Read the model definition and answer for the solid it produces. Units are mm, in the model's axes. A direction names the side the tool comes from. Coordinates: 2 decimals unless noted, no trailing zeros. Write each loop counter-clockwise with the first axis right and the second up, starting at its lowest first coordinate (ties: lowest second). Pieces come first, ordered by that corner, then holes.
Item 1: Each of these flat-tipped pins is pushed along its axis until it touches: P1, Ø4.5, axis at x = -9, z = -9.5, coming from the -Y side; P2, Ø18, axis at x = -47, z = -8, coming from the -Y side; P3, Ø10, axis at x = -26.5, y = 9.5, coming from the +Z side; P4, Ø2, axis at y = 11.5, z = -3, coming from the -X side. Where does it stop, or does it pass through?
Item 2: Straight lines are drawn through the part: probe 1 along Y at (x, z) = (-68, 11); probe 2 along Z at (x, y) = (7, 49.5); probe 3 along Y at (x, z) = (16, 2.5). For each, find the intervals that lie inside material, in ascending order.
Item 3: A tool of negligible diameter and unlimited length cuts with its end or side. For faces 4 (the face through (23, 30, -29)), 5 (the face through (-25, 47, 0)), 6 (the face through (-61.466, 57.479, -10.082)), 7 (the face through (7.5, 46.5, 10.7)), 8 (the face through (20, 6, 0)), from which of +Z, -Z, +X, -X, +Y, -Y can it reach the whole face along a straight path? Write none if from no direction.
Item 4: Determine the mould class of faces 1 (the face through (-51.5, 62, -14)), 2 (the face through (1, 80, 28)), 3 (the face through (23, 1, -19)) for opening direction Z: released by +Z, released by -Z, zero draft, split by the parting line, or undercut.
Item 5: Section A-A (x = -16.5) is taken. Give the vertices of the cut face in (y, z) (3 decimals).
Item 6: Section C-C (y = 39) is taken. Give the vertices of the cut face in (x, z) (3 decimals), then the cut area to 3 significant figures.
Item 7: Section D-D (x = 81) is taken. Give the vertices of the cut face in (y, z).
Item 8: Section B-B (z = 19) is taken. Give the vertices of the cut face in (x, y).
from build123d import *

# Parameters (mm, degrees)
BOSS_EXTRUDE1_DEPTH            = 30
BOSS_EXTRUDE1_DEPTH_BACK       = 30
CUT_REVOLVE2_START             = 59
CUT_REVOLVE2_DEPTH             = 7
CUT_REVOLVE2_START_2           = 56
CUT_REVOLVE2_2_DEPTH           = 3
CUT_EXTRUDE1_DEPTH             = 22.615
CUT_EXTRUDE2_REACH             = 143.287
CUT_EXTRUDE2_DIRECTION_2_DEPTH = 142.286942072
FILLET5_R                      = 5
FILLET6_R                      = 5
SKETCH7_W                      = 18.23
SKETCH7_H                      = 1.85
CUT_EXTRUDE3_DEPTH             = 17.32
SKETCH8_W                      = 20
SKETCH8_H                      = 24.63
CUT_EXTRUDE4_DEPTH             = 15.3
CUT_EXTRUDE5_REACH             = 133.385
SKETCH10_R                     = 1
SKETCH12_R                     = 2.5
CUT_EXTRUDE6_DEPTH             = 10.5
CUT_EXTRUDE7_REACH             = 133.385
SKETCH13_R                     = 1
SKETCH14_R                     = 2.5
CUT_EXTRUDE8_DEPTH             = 34.5


# Read off the part's stored shape, not the designer's step: Cut-Revolve2
with BuildPart() as part:
    # Sketch1 → Boss-Extrude1 (new, two sides: drawn at the far end of the back side and taken through both)
    with BuildSketch(Plane.XY.offset(-BOSS_EXTRUDE1_DEPTH_BACK)):
        Polygon((-25, 0), (-25, 56), (-99, 56), (-99, 81), (99, 81), (99, 56), (25, 56), (25, 0), align=None)
    extrude(amount=BOSS_EXTRUDE1_DEPTH + BOSS_EXTRUDE1_DEPTH_BACK)

    # Cut-Revolve2 outline → Cut-Revolve2 (cut)
    with BuildSketch(Plane(origin=(0, 0, 0), x_dir=(1, 0, 0), z_dir=(0, 1, 0)).offset(CUT_REVOLVE2_START)):
        with BuildLine():
            ThreePointArc((-37.5, -6), (-43.043277195, -2.296100594), (-41.742640687, 4.242640687))
            Line((-41.742640687, 4.242640687), (-61.54163056, 24.04163056))
            ThreePointArc((-61.54163056, 24.04163056), (-71.129711609, -5.004247907), (-53.5, -30))
            Line((-53.5, -30), (-37.5, -30))
            Line((-37.5, -30), (-37.5, -6))
        make_face()
    cut_revolve2 = extrude(amount=CUT_REVOLVE2_DEPTH, mode=Mode.SUBTRACT)

    # Cut-Revolve2 2 outline → Cut-Revolve2 2 (cut)
    with BuildSketch(Plane(origin=(0, 0, 0), x_dir=(1, 0, 0), z_dir=(0, 1, 0)).offset(CUT_REVOLVE2_START_2)):
        with BuildLine():
            Line((-37.5, -26), (-37.5, -14))
            ThreePointArc((-37.5, -14), (-50.434313455, -5.357568053), (-47.399494937, 9.899494937))
            Line((-47.399494937, 9.899494937), (-55.884776311, 18.384776311))
            ThreePointArc((-55.884776311, 18.384776311), (-61.520867845, -9.949769241), (-37.5, -26))
        make_face()
    cut_revolve2_2 = extrude(amount=CUT_REVOLVE2_2_DEPTH, mode=Mode.SUBTRACT)

    # Sketch4 → Cut-Extrude1 (cut)
    with BuildSketch(Plane.ZY.offset(25)):
        Polygon((12.315, 12.5), (-12.315, 12.5), (-12.315, 44.5), (-6.965, 44.5), (-6.965, 45.65), (7.015, 45.65), (7.015, 44.5), (12.315, 44.5), align=None)
    cut_extrude1 = extrude(amount=-CUT_EXTRUDE1_DEPTH, mode=Mode.SUBTRACT)

    # Mirror1: Cut-Extrude1 across plane
    add(cut_extrude1.mirror(Plane.ZY), mode=Mode.SUBTRACT)

    # Sketch5 → Cut-Extrude2 (cut, up to next)
    with BuildSketch(Plane.XY.offset(30), mode=Mode.PRIVATE) as cut_extrude2_sk1:
        Polygon((-63.5, 56), (-37.5, 56), (-37.5, 66), (-71.5, 66), (-71.5, 59), (-63.5, 59), align=None)
    cut_extrude2_tool1 = extrude(cut_extrude2_sk1.sketch, amount=-CUT_EXTRUDE2_REACH, mode=Mode.PRIVATE) & part.part
    cut_extrude2 = cut_extrude2_tool1.solids().sort_by_distance((-53.512658, 61.265823, 30))[0]
    add(cut_extrude2, mode=Mode.SUBTRACT)

    # Sketch5 → Cut-Extrude2 direction 2 (cut)
    with BuildSketch(Plane.XY.offset(30)):
        Polygon((-63.5, 56), (-37.5, 56), (-37.5, 66), (-71.5, 66), (-71.5, 59), (-63.5, 59), align=None)
    cut_extrude2_direction_2 = extrude(amount=CUT_EXTRUDE2_DIRECTION_2_DEPTH, mode=Mode.SUBTRACT)

    # Mirror4: Cut-Revolve2, Cut-Revolve2 2 across plane
    add(cut_revolve2.mirror(Plane.ZY), mode=Mode.SUBTRACT)
    add(cut_revolve2_2.mirror(Plane.ZY), mode=Mode.SUBTRACT)

    # Mirror2: Cut-Extrude2, Cut-Extrude2 direction 2 across plane
    add(cut_extrude2.mirror(Plane.ZY), mode=Mode.SUBTRACT)
    add(cut_extrude2_direction_2.mirror(Plane.ZY), mode=Mode.SUBTRACT)

    # Fillet5
    fillet5_edges = [part.edges().sort_by_distance(p)[0] for p in [
        (-99, 81, 0),
        (99, 81, 0),
        (0, 81, -30),
        (0, 81, 30),
    ]]
    fillet(fillet5_edges, radius=FILLET5_R)

    # Fillet6
    fillet6_edges = [part.edges().sort_by_distance(p)[0] for p in [
        (-25, 0, 0),
        (-99, 56, 0),
        (99, 56, 0),
        (25, 0, 0),
        (0, 0, 30),
        (25, 28, 30),
        (-25, 28, 30),
        (-25, 28, -30),
        (0, 0, -30),
        (25, 28, -30),
    ]]
    fillet(fillet6_edges, radius=FILLET6_R)

    # Sketch7 → Cut-Extrude3 (cut)
    with BuildSketch(Plane.ZY.offset(25)):
        with Locations((0, 11.575)):
            Rectangle(SKETCH7_W, SKETCH7_H)
    cut_extrude3 = extrude(amount=-CUT_EXTRUDE3_DEPTH, mode=Mode.SUBTRACT)

    # Mirror5: Cut-Extrude3 across plane
    add(cut_extrude3.mirror(Plane.ZY), mode=Mode.SUBTRACT)

    # Sketch8 → Cut-Extrude4 (cut)
    with BuildSketch(Plane.XZ):
        with Locations((-30, 0)):
            Rectangle(SKETCH8_W, SKETCH8_H)
        with Locations((30, 0)):
            Rectangle(SKETCH8_W, SKETCH8_H)
    extrude(amount=-CUT_EXTRUDE4_DEPTH, mode=Mode.SUBTRACT)

    # Sketch10 → Cut-Extrude5 (cut, up to next)
    with BuildSketch(Plane(origin=(0, 0, 0), x_dir=(-1, 0, 0), z_dir=(0, -1, 0)), mode=Mode.PRIVATE) as cut_extrude5_sk1:
        with Locations(Location((4.785, -10.165, 0), (0, 0, 90))):
            Circle(SKETCH10_R)
    cut_extrude5_tool1 = extrude(cut_extrude5_sk1.sketch, amount=-CUT_EXTRUDE5_REACH, mode=Mode.PRIVATE) & part.part
    # Sketch10 → Cut-Extrude5 (cut, up to next)
    with BuildSketch(Plane(origin=(0, 0, 0), x_dir=(-1, 0, 0), z_dir=(0, -1, 0)), mode=Mode.PRIVATE) as cut_extrude5_sk2:
        with Locations(Location((4.785, 10.165, 0), (0, 0, 180))):
            Circle(SKETCH10_R)
    cut_extrude5_tool2 = extrude(cut_extrude5_sk2.sketch, amount=-CUT_EXTRUDE5_REACH, mode=Mode.PRIVATE) & part.part
    # Sketch10 → Cut-Extrude5 (cut, up to next)
    with BuildSketch(Plane(origin=(0, 0, 0), x_dir=(-1, 0, 0), z_dir=(0, -1, 0)), mode=Mode.PRIVATE) as cut_extrude5_sk3:
        with Locations(Location((-4.785, 10.165, 0), (0, 0, 90))):
            Circle(SKETCH10_R)
    cut_extrude5_tool3 = extrude(cut_extrude5_sk3.sketch, amount=-CUT_EXTRUDE5_REACH, mode=Mode.PRIVATE) & part.part
    # Sketch10 → Cut-Extrude5 (cut, up to next)
    with BuildSketch(Plane(origin=(0, 0, 0), x_dir=(-1, 0, 0), z_dir=(0, -1, 0)), mode=Mode.PRIVATE) as cut_extrude5_sk4:
        with Locations((-4.785, -10.165)):
            Circle(SKETCH10_R)
    cut_extrude5_tool4 = extrude(cut_extrude5_sk4.sketch, amount=-CUT_EXTRUDE5_REACH, mode=Mode.PRIVATE) & part.part
    add(cut_extrude5_tool1.solids().sort_by_distance((-4.785, 0, 10.165))[0], mode=Mode.SUBTRACT)
    add(cut_extrude5_tool2.solids().sort_by_distance((-4.785, 0, -10.165))[0], mode=Mode.SUBTRACT)
    add(cut_extrude5_tool3.solids().sort_by_distance((4.785, 0, -10.165))[0], mode=Mode.SUBTRACT)
    add(cut_extrude5_tool4.solids().sort_by_distance((4.785, 0, 10.165))[0], mode=Mode.SUBTRACT)

    # Sketch12 → Cut-Extrude6 (cut)
    with BuildSketch(Plane.XZ):
        with Locations(Location((-4.785, 10.165, 0), (0, 0, 270))):
            Circle(SKETCH12_R)
        with Locations((-4.785, -10.165)):
            Circle(SKETCH12_R)
        with Locations(Location((4.785, -10.165, 0), (0, 0, 270))):
            Circle(SKETCH12_R)
        with Locations((4.785, 10.165)):
            Circle(SKETCH12_R)
    extrude(amount=-CUT_EXTRUDE6_DEPTH, mode=Mode.SUBTRACT)

    # Sketch13 → Cut-Extrude7 (cut, up to next)
    with BuildSketch(Plane(origin=(0, 81, 0), x_dir=(1, 0, 0), z_dir=(0, 1, 0)), mode=Mode.PRIVATE) as cut_extrude7_sk1:
        with Locations(Location((-8.585, 10.165, 0), (0, 0, 270))):
            Circle(SKETCH13_R)
    cut_extrude7_tool1 = extrude(cut_extrude7_sk1.sketch, amount=-CUT_EXTRUDE7_REACH, mode=Mode.PRIVATE) & part.part
    # Sketch13 → Cut-Extrude7 (cut, up to next)
    with BuildSketch(Plane(origin=(0, 81, 0), x_dir=(1, 0, 0), z_dir=(0, 1, 0)), mode=Mode.PRIVATE) as cut_extrude7_sk2:
        with Locations(Location((-8.585, -10.165, 0), (0, 0, 180))):
            Circle(SKETCH13_R)
    cut_extrude7_tool2 = extrude(cut_extrude7_sk2.sketch, amount=-CUT_EXTRUDE7_REACH, mode=Mode.PRIVATE) & part.part
    # Sketch13 → Cut-Extrude7 (cut, up to next)
    with BuildSketch(Plane(origin=(0, 81, 0), x_dir=(1, 0, 0), z_dir=(0, 1, 0)), mode=Mode.PRIVATE) as cut_extrude7_sk3:
        with Locations(Location((8.585, -10.165, 0), (0, 0, 270))):
            Circle(SKETCH13_R)
    cut_extrude7_tool3 = extrude(cut_extrude7_sk3.sketch, amount=-CUT_EXTRUDE7_REACH, mode=Mode.PRIVATE) & part.part
    # Sketch13 → Cut-Extrude7 (cut, up to next)
    with BuildSketch(Plane(origin=(0, 81, 0), x_dir=(1, 0, 0), z_dir=(0, 1, 0)), mode=Mode.PRIVATE) as cut_extrude7_sk4:
        with Locations((8.585, 10.165)):
            Circle(SKETCH13_R)
    cut_extrude7_tool4 = extrude(cut_extrude7_sk4.sketch, amount=-CUT_EXTRUDE7_REACH, mode=Mode.PRIVATE) & part.part
    add(cut_extrude7_tool1.solids().sort_by_distance((-8.585, 81, -10.165))[0], mode=Mode.SUBTRACT)
    add(cut_extrude7_tool2.solids().sort_by_distance((-8.585, 81, 10.165))[0], mode=Mode.SUBTRACT)
    add(cut_extrude7_tool3.solids().sort_by_distance((8.585, 81, 10.165))[0], mode=Mode.SUBTRACT)
    add(cut_extrude7_tool4.solids().sort_by_distance((8.585, 81, -10.165))[0], mode=Mode.SUBTRACT)

    # Sketch14 → Cut-Extrude8 (cut)
    with BuildSketch(Plane(origin=(0, 81, 0), x_dir=(1, 0, 0), z_dir=(0, 1, 0))):
        with Locations(Location((-8.585, 10.165, 0), (0, 0, 270))):
            Circle(SKETCH14_R)
        with Locations(Location((-8.585, -10.165, 0), (0, 0, 180))):
            Circle(SKETCH14_R)
        with Locations(Location((8.585, -10.165, 0), (0, 0, 270))):
            Circle(SKETCH14_R)
        with Locations(Location((8.585, 10.165, 0), (0, 0, 180))):
            Circle(SKETCH14_R)
    extrude(amount=-CUT_EXTRUDE8_DEPTH, mode=Mode.SUBTRACT)


solid = part.part
Established:
1. P1: stops at y = 0
1. P2: stops at y = 56
1. P3: stops at z = 29.77
1. P4: stops at x = -20
2. probe 1: y = 56 to 59, 66 to 81
2. probe 2: z = -30 to -12.1, -8.23 to 8.23, 12.1 to 30
2. probe 3: y = 0 to 10.65, 45.65 to 81
3. face 4: -Z, +X, -Y
3. face 5: +Z, -Z, -X, -Y
3. face 6: +Z, -Y
3. face 7: +Y
3. face 8: +X, -Y
4. face 1: undercut
4. face 2: released by +Z
4. face 3: zero draft
5. outline: (0, -25) arc R5 ccw to (5, -30) - (76, -30) arc R5 ccw to (81, -25) - (81, 25) arc R5 ccw to (76, 30) - (5, 30) arc R5 ccw to (0, 25) - close; hole (10.65, -9.115) - (12.5, -9.115) - (12.5, -12.315) - (44.5, -12.315) - (44.5, -6.965) - (45.65, -6.965) - (45.65, 7.015) - (44.5, 7.015) - (44.5, 12.315) - (12.5, 12.315) - (12.5, 9.115) - (10.65, 9.115) - close
6. outline: (-25, -25) arc R5 ccw to (-20, -30) - (20, -30) arc R5 ccw to (25, -25) - (25, -12.315) - (2.385, -12.315) - (2.385, 12.315) - (25, 12.315) - (25, 25) arc R5 ccw to (20, 30) - (-20, 30) arc R5 ccw to (-25, 25) - (-25, 12.315) - (-2.385, 12.315) - (-2.385, -12.315) - (-25, -12.315) - close
6. area: 1,860 mm2
7. outline: (56, -30) - (76, -30) arc R5 ccw to (81, -25) - (81, 25) arc R5 ccw to (76, 30) - (56, 30) - close
8. outline: (-99, 61) arc R5 ccw to (-94, 56) - (-63.5, 56) - (-63.5, 59) - (-71.5, 59) - (-71.5, 66) - (-37.5, 66) - (-37.5, 56) - (-25, 56) - (-25, 5) arc R5 ccw to (-20, 0) - (20, 0) arc R5 ccw to (25, 5) - (25, 56) - (37.5, 56) - (37.5, 66) - (71.5, 66) - (71.5, 59) - (63.5, 59) - (63.5, 56) - (94, 56) arc R5 ccw to (99, 61) - (99, 76) arc R5 ccw to (94, 81) - (-94, 81) arc R5 ccw to (-99, 76) - close
